```python
from build123d import *

# Parameters (mm, degrees)
SKETCH_R     = 4.7625
SKETCH_R_2   = 3.175
PAD_DEPTH    = 26
POCKET_DEPTH = 2.54
CHAMFER_SIZE = 0.5


with BuildPart() as part:
    # Sketch → Pad (new body)
    with BuildSketch(Plane.XY):
        Circle(SKETCH_R)
        Circle(SKETCH_R_2, mode=Mode.SUBTRACT)
    extrude(amount=PAD_DEPTH)

    # Sketch001 (on Face4 of Pad) → Pocket (cut)
    with BuildSketch(Plane.XY.offset(26)):
        with BuildLine():
            Line((1.15, 4.943999), (1.15, 2.567225))
            ThreePointArc((-1.15, 2.567225), (0, -2.813031), (1.15, 2.567225))
            Line((-1.15, 2.567225), (-1.15, 4.943999))
            ThreePointArc((-1.15, 4.943999), (0, -5.075985), (1.15, 4.943999))
        make_face()
    extrude(amount=-POCKET_DEPTH, mode=Mode.SUBTRACT)

    # Sketch002 → Groove (revolve, cut)
    with BuildSketch(Plane.YZ):
        with BuildLine():
            ThreePointArc((3.65, 25.944313), (2.65, 26.944313), (1.65, 25.944313))
            Line((1.65, 25.944313), (1.65, 23))
            ThreePointArc((1.65, 23), (2.65, 22), (3.65, 23))
            Line((3.65, 23), (3.65, 25.944313))
        make_face()
    revolve(axis=Axis((0, 0, 0), (0, 0, 1)), mode=Mode.SUBTRACT)

    # Chamfer
    chamfer_edges = [part.edges().sort_by_distance(p)[0] for p in [
        (-4.7625, 0, 0),
        (-3.175, 0, 0),
    ]]
    chamfer(chamfer_edges, length=CHAMFER_SIZE)


solid = part.part
```
Here's how the part is built. I have some questions about the finished solid (model axes, mm). A direction names the side the tool comes from. Give positions to 0.01 mm unless a question says otherwise; leave off trailing zeros. Put each result on its own line as item: value. Start each with the question number.
Item 1: Thinking about a two-plate mould opening in Y: for faces 4 (the cylindrical face through (0.48, 3.62, 23.61)), 5 (the cylindrical face through (-2.52, -1.93, 11.17)), 6 (the cylindrical face through (-0.62, 4.72, 13.07)), 7 (the flat face through (0, 4, 26)), which applies, +Y half, -Y half, draft (parallel to the pull), parting line (faces both ways), or undercut?
Item 2: I need wall thicknesses on L1, parallel to X at y = 0, z = 16.25 (1 decimal); L2, parallel to Z at x = 3.25, y = -2.5. Which ranges of each line are inside material? Lowest first, please. Write a range as from..to.
Item 3: On a 3-axis mill with a long thin cutter (end or side, diameter ignored), from which of +Z, -Z, +X, -X, +Y, -Y can I reach the whole of each face in a straight line? I mean faces 1 (the flat face through (0, 4, 0)), 2 (the flat face through (-1.15, 4, 25)), 3 (the flat face through (1.15, 4, 25)). Say none if no direction works.
Item 4: Will these pins go through, and if not, where does the flat tip stop? pin 1 (1 mm diameter, centred on y = 1.5, z = 15, fed in from -X); pin 2 (0.6 mm diameter, centred on y = 4, z = 25, fed in from +X); pin 3 (1.5 mm diameter, centred on y = 2, z = 14, fed in from -X).
Values:
1. face 4: undercut
1. face 5: undercut
1. face 6: parting line
1. face 7: draft
2. L1: -4.8..-3.2, 3.2..4.8
2. L2: 0..23.46
3. face 1: -Z, +X, -X, +Y, -Y
3. face 2: +Z, -X, +Y, -Y
3. face 3: +Z, +X, +Y, -Y
4. pin 1: x = -4.66
4. pin 2: x = 1.15
4. pin 3: x = -4.6
